from build123d import *

# Parameters (mm, degrees)
F1_DEPTH = 63.5
F2_DEPTH = 25.4
F3_DEPTH = 7.9375
F0_W     = 25.4
F0_H     = 19.05
F0_H_2   = 4.7752
F0_H_3   = 4.7498
F5_R     = 6.35


with BuildPart() as f1:
    # F0 (on Front) → F1 (new body, symmetric)
    with BuildSketch(Plane.XZ):
        Polygon((41.275, -6.35), (41.275, 6.35), (22.225, 6.35), (-41.275, 6.35), (-41.275, -6.35), align=None)
    extrude(amount=F1_DEPTH, both=True)

    # F0 (on Front) → F2 (join, symmetric)
    with BuildSketch(Plane.XZ):
        with BuildLine():
            Line((22.225, 6.35), (41.275, 6.35))
            Line((41.275, 6.35), (41.275, 30.1752))
            ThreePointArc((41.275, 30.1752), (45.9246798487, 41.4005201513), (57.15, 46.0502))
            Line((57.15, 46.0502), (68.3291607261, 46.0502))
            Line((68.3291607261, 46.0502), (68.3291607261, 65.1002))
            Line((68.3291607261, 65.1002), (57.15, 65.1002))
            add(Edge.make_bspline(
                [(57.15, 65.1002), (56.2738590878, 65.0736826773), (55.4037055369, 65.041136828), (54.5394513338, 65.0024976365)],
                knots=[0, 0, 0, 0, 2.264919631, 2.264919631, 2.264919631, 2.264919631], degree=3))
            ThreePointArc((54.5394513338, 65.0024976365), (31.5479587028, 53.9300122791), (22.225, 30.1752))
            Line((22.225, 30.1752), (22.225, 6.35))
        make_face()
    extrude(amount=F2_DEPTH, both=True)

    # F0 (on Front) → F3 (join, symmetric)
    with BuildSketch(Plane.XZ):
        with BuildLine():
            Line((-41.275, 6.35), (22.225, 6.35))
            Line((22.225, 6.35), (22.225, 30.1752))
            ThreePointArc((22.225, 30.1752), (31.5479587028, 53.9300122791), (54.5394513338, 65.0024976365))
            add(Edge.make_bspline(
                [(54.5394513338, 65.0024976365), (11.6644928166, 63.085638308), (-16.6917426365, 46.172621582), (-41.275, 6.35)],
                knots=[2.264919631, 2.264919631, 2.264919631, 2.264919631, 114.6257677184, 114.6257677184, 114.6257677184, 114.6257677184], degree=3))
        make_face()
    extrude(amount=F3_DEPTH, both=True)

    # F0 (on Front) → F4 (revolve)
    with BuildSketch(Plane.XZ):
        with Locations((81.0291607261, 55.5752)):
            Rectangle(F0_W, F0_H)
        with Locations((81.0291607261, 43.6626)):
            Rectangle(F0_W, F0_H_2)
        with Locations((81.0291607261, 67.4751)):
            Rectangle(F0_W, F0_H_3)
    revolve(axis=Axis((68.3291607261, 0, 55.5625), (0, 0, -1)))

    # F5
    f5_edges = [f1.edges().sort_by_distance(p)[0] for p in [
        (41.275, -63.5, 0),
        (41.275, 63.5, 0),
        (-41.275, -63.5, 0),
        (-41.275, 63.5, 0),
    ]]
    fillet(f5_edges, radius=F5_R)


solid = f1.part
Verification items for the finished model (mm, model axes). A direction names the side the tool comes from. Coordinates: 2 decimals unless noted, no trailing zeros. Loops run counter-clockwise (first coordinate to the right, second up) from the corner with the lowest first, then second, coordinate; pieces in that order, holes last. Notation, with made-up numbers: (18, -39.5) -> (40, -39.5) arc R28 ccw to (40, -17.5) -> close; hole circle Ø3 at (89, 63). An arc over 180 degrees is marked (long way). Answer as CSV lines item,"result".
1) Thickness scan on L1, parallel to Z at x = -30.5, y = 44; L2, parallel to Y at x = 2, z = 41; L3, parallel to X at y = -39, z = 1 (3 decimals). Record the ranges inside material, lowest first. Write a range as from..to.
Found:
L1,"z = -6.35..6.35"
L2,"y = -7.94..7.94"
L3,"x = -41.275..41.275"
2) Cross-section at A-A, the plane y = 38.5. Record the cut outline in (x, z) (3 decimals), then the cut area to 3 significant figures.
Found:
outline,"(-41.275, -6.35) -> (41.275, -6.35) -> (41.275, 6.35) -> (-41.275, 6.35) -> close"
area,"1,050 mm2"
3) Tool access check on faces 1 (the cylindrical face through (31.8, 16.5, 54.2)), 2 (the flat face through (40, 25.4, 36)), 3 (the flat face through (70, 0, 41.275)), 4 (the flat face through (1, -7.938, 29)), 5 (the flat face through (40, -25.4, 36)). Record the directions out of +Z, -Z, +X, -X, +Y, -Y that give a thin tool (end or side, any length) a straight path to the whole face; none if there is none.
Found:
face 1,"+Z, -X, +Y"
face 2,"+Z, +X, -X, +Y"
face 3,"-Z, +X, +Y, -Y"
face 4,"+Z, -X, -Y"
face 5,"+Z, +X, -X, -Y"
4) Depth check by flat-ended pin: pin 1 (1.5 mm diameter, centred on x = -19.5, z = 38, fed in from -Y); pin 2 (23 mm diameter, centred on x = 37.5, z = 30.5, fed in from +Y); pin 3 (1.3 mm diameter, centred on x = 60.5, y = -24, fed in from -Z) (3 decimals); pin 4 (3 mm diameter, centred on y = 42.5, z = 3, fed in from +X) (3 decimals). Enter the tip coordinate at first touch or a pass-through.
Found:
pin 1,"passes through"
pin 2,"stops at y = 25.4"
pin 3,"stops at z = 41.275"
pin 4,"stops at x = 41.275"
5) Cross-section at B-B, the plane x = 75.5. Record the cut outline in (y, z) (3 decimals), then the cut area to 3 significant figures.
Found:
outline,"(-24.367, 41.275) -> (24.367, 41.275) -> (24.367, 69.85) -> (-24.367, 69.85) -> close"
area,"1,390 mm2"
